Here's how the part is built. I have some questions about the finished solid (model axes, mm). Round coordinates to 2 decimals unless told otherwise and drop trailing zeros. Write each loop counter-clockwise with the first axis right and the second up, starting at its lowest first coordinate (ties: lowest second). Pieces come first, ordered by that corner, then holes. Notation, with made-up numbers: (-10.75, 75) - (28.25, 75) arc R18 cw to (28.25, 104) - close; hole circle Ø9 at (28, 10). An arc over 180 degrees is marked (long way). Use one line per item in the form item = value. Start each with the question number.
1. I want a section at A-A, the plane y = -111. List the corners of the cut face in (x, z) for me, plus the area to 3 significant figures.
2. Will these pins go through, and if not, where does the flat tip stop? pin 1 (1.8 mm diameter, centred on x = 809, z = 1.5, fed in from +Y); pin 2 (1.5 mm diameter, centred on y = -325.5, z = 0.5, fed in from +X); pin 3 (1.8 mm diameter, centred on y = -357.5, z = 4.5, fed in from -X).
3. If I drill on line 1 along X through (y, z) = (-520.7, 2.1); line 2 along Y through (x, z) = (800.1, 4.85); line 3 along X through (y, z) = (-342, 4.4), over which ranges is the centre line in solid material (lowest first)?
```python
from build123d import *

# Parameters (mm, degrees)
SKETCH_R      = 3.9751
EXTRUDE_DEPTH = 5.9944


with BuildPart() as part:
    # Sketch → Extrude (new body)
    with BuildSketch(Plane.XY):
        with BuildLine():
            Line((0, 0), (0, -50.8))
            Line((0, -50.8), (8.7249, -50.8))
            Line((8.7249, -50.8), (8.7249, -38.1))
            ThreePointArc((16.6751, -38.1), (12.7, -34.1249), (8.7249, -38.1))
            Line((16.6751, -38.1), (16.6751, -495.3))
            ThreePointArc((8.7249, -495.3), (12.7, -499.2751), (16.6751, -495.3))
            Line((8.7249, -495.3), (8.7249, -482.6))
            Line((8.7249, -482.6), (0, -482.6))
            Line((0, -482.6), (0, -533.4))
            Line((0, -533.4), (812.8, -533.4))
            Line((812.8, -533.4), (812.8, -482.6))
            Line((812.8, -482.6), (804.0751, -482.6))
            Line((804.0751, -482.6), (804.0751, -495.3))
            ThreePointArc((796.1249, -495.3), (800.1, -499.2751), (804.0751, -495.3))
            Line((796.1249, -38.1), (796.1249, -495.3))
            ThreePointArc((804.0751, -38.1), (800.1, -34.1249), (796.1249, -38.1))
            Line((804.0751, -50.8), (804.0751, -38.1))
            Line((812.8, -50.8), (804.0751, -50.8))
            Line((812.8, 0), (812.8, -50.8))
            Line((0, 0), (812.8, 0))
        make_face()
        with Locations((12.7, -12.7)):
            Circle(SKETCH_R, mode=Mode.SUBTRACT)
        with Locations((800.1, -12.7)):
            Circle(SKETCH_R, mode=Mode.SUBTRACT)
        with Locations((12.7, -520.7)):
            Circle(SKETCH_R, mode=Mode.SUBTRACT)
        with Locations((800.1, -520.7)):
            Circle(SKETCH_R, mode=Mode.SUBTRACT)
    extrude(amount=EXTRUDE_DEPTH)


solid = part.part
```
Model answer:
q1.outline = (16.68, 0) - (796.12, 0) - (796.12, 5.99) - (16.68, 5.99) - close
q1.area = 4,670 mm2
q2.pin_1 = 0
q2.pin_2 = 796.12
q2.pin_3 = 16.68
q3.line_1 = 0 to 8.72, 16.68 to 796.12, 804.08 to 812.8
q3.line_2 = -533.4 to -524.68, -516.72 to -499.28, -34.12 to -16.68, -8.72 to 0
q3.line_3 = 16.68 to 796.12
